Verification items for the finished model (mm, model axes). Coordinates: 2 decimals unless noted, no trailing zeros. Loops run counter-clockwise (first coordinate to the right, second up) from the corner with the lowest first, then second, coordinate; pieces in that order, holes last. Notation, with made-up numbers: (80.5, 49) -> (130.5, 49) arc R29 cw to (130.5, 77) -> close; hole circle Ø6 at (16.25, 64). An arc over 180 degrees is marked (long way). Write item = value, one per line.
```python
from build123d import *

# Parameters (mm, degrees)
F1_R           = 17
F2_DEPTH       = 19
F4_D           = 3
F4_CSINK_D     = 8
F4_CSINK_ANGLE = 90
F5_D           = 4.4


with BuildPart() as f2:
    # F1 (on Front) → F2 (new body)
    with BuildSketch(Plane.XZ):
        Polygon((105, 0), (105, 220), (0, 325), (-105, 220), (-105, 0), align=None)
        with Locations((0, 140)):
            Circle(F1_R, mode=Mode.SUBTRACT)
    extrude(amount=F2_DEPTH)

    # F4 (through all)
    with Locations(Plane.XZ.offset(19)):
        with Locations((95.5, 25), (95.5, 115), (95.5, 205), (-76.5, 175)):
            CounterSinkHole(F4_D / 2, F4_CSINK_D / 2, counter_sink_angle=F4_CSINK_ANGLE)

    # F5 (through all)
    with Locations(Plane.XZ.offset(19)):
        with Locations((-95.5, 210.5)):
            Hole(F5_D / 2)


solid = f2.part
```
1) Material ranges on line 1 (Z direction, x = 96, y = -2.5); line 2 (X direction, y = -6.75, z = 175); line 3 (Z direction, x = 95.5, y = -12.5), recorded low to high.
Ans:
line_1 = 0 to 23.59, 26.41 to 113.59, 116.41 to 203.59, 206.41 to 229
line_2 = -105 to -78, -75 to 105
line_3 = 0 to 23.5, 26.5 to 113.5, 116.5 to 203.5, 206.5 to 229.5
2) Sectioned sample at A-A, the plane x = 13. Record the cut outline in (y, z), plus the area to 3 significant figures.
Ans:
outline = (-19, 0) -> (0, 0) -> (0, 129.05) -> (-19, 129.05) -> close; (-19, 150.95) -> (0, 150.95) -> (0, 312) -> (-19, 312) -> close
area = 5,510 mm2
3) Release check for a two-part mould opening along Z. For faces 1 (the face through (105, -9, 108)), 2 (the face through (93.953, -16.621, 25.487)), 3 (the face through (-1, -9, 0)) record: pulls with the +Z half, pulls with the -Z half, needs draft (parallel to the pull), parting line crosses it, or undercut.
Ans:
face_1 = needs draft
face_2 = undercut
face_3 = pulls with the -Z half
4) Sectioned sample at B-B, the plane y = -10.5. Record the cut outline in (x, z), plus the area to 3 significant figures.
Ans:
outline = (-105, 0) -> (105, 0) -> (105, 220) -> (0, 325) -> (-105, 220) -> close; hole circle Ø4.4 at (-95.5, 210.5); hole circle Ø3 at (-76.5, 175); hole circle Ø34 at (0, 140); hole circle Ø3 at (95.5, 25); hole circle Ø3 at (95.5, 115); hole circle Ø3 at (95.5, 205)
area = 56,300 mm2
5) Depth check by flat-ended pin: pin 1 Ø4 at (x, z) = (82.5, 175) entering from +Y; pin 2 Ø2.5 at (x, z) = (95.5, 205) entering from -Y; pin 3 Ø10 at (y, z) = (-10.5, 287.5) entering from -X; pin 4 Ø2 at (x, y) = (67.5, -10) entering from +Z. Enter the tip coordinate at first touch or a pass-through.
Ans:
pin_1 = 0
pin_2 = through
pin_3 = -42.5
pin_4 = 258.5
6) Sectioned sample at D-D, the plane x = -27.5. Record the cut outline in (y, z), plus the area to 3 significant figures.
Ans:
outline = (-19, 0) -> (0, 0) -> (0, 297.5) -> (-19, 297.5) -> close
area = 5,650 mm2
7) Sectioned sample at C-C, the plane z = 282.5. Record the cut outline in (x, y).
Ans:
outline = (-42.5, -19) -> (42.5, -19) -> (42.5, 0) -> (-42.5, 0) -> close
